Model file for the job. Use its own axes, mm. Round coordinates to 2 decimals unless told otherwise and drop trailing zeros. Order: outer loops, then holes, each group sorted by start corner. A loop starts at its lowest first (then second) coordinate and runs counter-clockwise, first axis right, second up. Notation, with made-up numbers: M 51.25,46.5 L 97.25,46.5 A32 cw 97.25,76.5 Z; hole C -29.75,-10 d11. An arc over 180 degrees is marked long. Return JSON: item names as keys, results as strings. Group by question number.
Item 1: Pin check, flat tips, straight feed: pin 1 Ø9 at (x, y) = (0, 27) entering from +Z; pin 2 Ø0.5 at (y, z) = (23.5, 0.5) entering from -X; pin 3 Ø9 at (x, y) = (0, 17.6) entering from -Z. Stop position of each tip, or through.
Item 2: Probe line 1 along X through (y, z) = (17.6, 0.3); line 2 along Y through (x, z) = (-0.25, 0.5); line 3 along X through (y, z) = (27, 0.6). List the from-to ranges inside material, lowest first.
Item 3: Pull direction Y, two halves, no side cores. Call faces 1 (the face through (-2.96, -34.9, 0.49)), 2 (the face through (0.206, 12.004, 0.493)), 3 (the face through (0.233, 35.497, 0.493)), 4 (the face through (0, 8, 1)): pulls with the +Y half, pulls with the -Y half, needs draft (parallel to the pull), parting line crosses it, or undercut.
Item 4: Slice it at C-C on z = 0.75. Write the cut outline in (x, y).
Item 5: Slice it at A-A on y = 17.6. Write the cut outline in (x, z).
Item 6: Slice it at D-D on y = -10.5. Write the cut outline in (x, z).
Item 7: Slice it at B-B on x = 0. Write the cut outline in (y, z).
from build123d import *

# Parameters (mm, degrees)
F2_DEPTH = 1


# Not quite as in the source:
# - ends of sketch curves that miss each other by under 0.0002 mm in the source are joined


with BuildPart() as f2:
    # F1 (on Top) → F2 (new body)
    with BuildSketch(Plane.XY):
        with BuildLine():
            Line((-1.534358, -35.5), (1.499849, -35.5))
            ThreePointArc((1.499849, -35.5), (2.9140625624, -34.9142135624), (3.499849, -33.5))
            Line((3.499849, -33.5), (3.499849, 5.24069))
            ThreePointArc((3.499849, 5.24069), (4.0745571603, 7.568090295), (5.6665658533, 9.3604602133))
            ThreePointArc((5.6665658533, 9.3604602133), (9.8857158615, 16.0924782241), (7.8648732423, 23.7760641903))
            ThreePointArc((7.8648732423, 23.7760641903), (1.896e-07, 35.5), (-7.8648736534, 23.7760641421))
            ThreePointArc((-7.8648736534, 23.7760641421), (-9.8878127884, 16.1062937833), (-5.6895721633, 9.376328764))
            ThreePointArc((-5.6895721633, 9.376328764), (-4.1058182159, 7.585707204), (-3.534358, 5.264493))
            Line((-3.534358, 5.264493), (-3.534358, -33.5))
            ThreePointArc((-3.534358, -33.5), (-2.9485715624, -34.9142135624), (-1.534358, -35.5))
        make_face()
        with BuildLine():
            Line((-2.729304, 22.489878), (-2.729304, 24.808904))
            ThreePointArc((-2.729304, 24.808904), (3.13e-07, 30.5), (2.7293033847, 24.8089036912))
            Line((2.7293033847, 24.8089036912), (2.729303, 22.489878))
            ThreePointArc((2.729303, 22.489878), (4.366e-07, 12), (-2.729304, 22.489878))
        make_face(mode=Mode.SUBTRACT)
    extrude(amount=F2_DEPTH)


solid = f2.part
Output values:
{
 "1": {"pin 1": "z = 1", "pin 2": "x = -8.25", "pin 3": "through"},
 "2": {"line 1": "-10 to -5.6, 5.6 to 10", "line 2": "-35.5 to 12.01, 30.49 to 35.5", "line 3": "-8.5 to -3.5, 3.5 to 8.5"},
 "3": {"face 1": "pulls with the -Y half", "face 2": "undercut", "face 3": "undercut", "face 4": "needs draft"},
 "4": {"outline": "M -7.86,23.78 A10 ccw -5.69,9.38 A5 cw -3.53,5.26 L -3.53,-33.5 A2 ccw -1.53,-35.5 L 1.5,-35.5 A2 ccw 3.5,-33.5 L 3.5,5.24 A5 cw 5.67,9.36 A10 ccw 7.86,23.78 A8.5 ccw long Z; hole M -2.73,22.49 A5.6 ccw long 2.73,22.49 L 2.73,24.81 A3.5 ccw long -2.73,24.81 Z"},
 "5": {"outline": "M -10,0 L -5.6,0 L -5.6,1 L -10,1 Z; M 5.6,0 L 10,0 L 10,1 L 5.6,1 Z"},
 "6": {"outline": "M -3.53,0 L 3.5,0 L 3.5,1 L -3.53,1 Z"},
 "7": {"outline": "M -35.5,0 L 12,0 L 12,1 L -35.5,1 Z; M 30.5,0 L 35.5,0 L 35.5,1 L 30.5,1 Z"}
}
